from build123d import *

# Parameters (mm, degrees)
SKETCH_1_R          = 2.5
EXTRUDE_1_DEPTH     = 47
EXTRUDE_START       = 47
SKETCH_2_R          = 4
EXTRUDE_2_DEPTH     = 49
EXTRUDE_START_2     = 96
SKETCH_3_R          = 5
EXTRUDE_3_DEPTH     = 3.5
EXTRUDE_START_3     = 99.5
SKETCH_4_R          = 4
EXTRUDE_4_DEPTH     = 18
EXTRUDE_START_4     = 2.2
EXTRUDE_5_DEPTH     = 3
CHAMFER_1_SIZE      = 0.25
CHAMFER_2_SIZE      = 0.1
CUT_EXTRUDE_START   = 117.5
SKETCH_6_R          = 1.5
CUT_EXTRUDE_1_DEPTH = 10


with BuildPart() as part:
    # 草图1 → 凸台-拉伸1 (new body)
    with BuildSketch(Plane(origin=(0, 0, 0), x_dir=(1, 0, 0), z_dir=(0, 1, 0))):
        with Locations(Location((0, 0, 0), (0, 0, 270))):
            Circle(SKETCH_1_R)
    extrude(amount=EXTRUDE_1_DEPTH)

    # 草图2 → 凸台-拉伸2 (add)
    with BuildSketch(Plane(origin=(0, 0, 0), x_dir=(1, 0, 0), z_dir=(0, 1, 0)).offset(EXTRUDE_START)):
        with Locations(Location((0, 0, 0), (0, 0, 270))):
            Circle(SKETCH_2_R)
    extrude(amount=EXTRUDE_2_DEPTH)

    # 草图3 → 凸台-拉伸3 (add)
    with BuildSketch(Plane(origin=(0, 0, 0), x_dir=(1, 0, 0), z_dir=(0, 1, 0)).offset(EXTRUDE_START_2)):
        with Locations(Location((0, 0, 0), (0, 0, 270))):
            Circle(SKETCH_3_R)
    extrude(amount=EXTRUDE_3_DEPTH)

    # 草图4 → 凸台-拉伸4 (add)
    with BuildSketch(Plane(origin=(0, 0, 0), x_dir=(1, 0, 0), z_dir=(0, 1, 0)).offset(EXTRUDE_START_3)):
        with Locations(Location((0, 0, 0), (0, 0, 270))):
            Circle(SKETCH_4_R)
    extrude(amount=EXTRUDE_4_DEPTH)

    # 草图11 → 凸台-拉伸5 (add)
    with BuildSketch(Plane.XY.offset(EXTRUDE_START_4)):
        with BuildLine():
            Line((-1.5, 103), (-1.5, 114))
            ThreePointArc((-1.5, 114), (0, 115.5), (1.5, 114))
            Line((1.5, 114), (1.5, 103))
            ThreePointArc((1.5, 103), (0, 101.5), (-1.5, 103))
        make_face()
    extrude(amount=EXTRUDE_5_DEPTH)

    # 倒角1
    chamfer_1_edges = [part.edges().sort_by_distance(p)[0] for p in [
        (0, 117.5, -4),
        (0, 0, -2.5),
    ]]
    chamfer(chamfer_1_edges, length=CHAMFER_1_SIZE)

    # 倒角2
    chamfer_2_edges = [part.edges().sort_by_distance(p)[0] for p in [
        (0, 101.5, 5.2),
        (1.5, 108.5, 5.2),
        (0, 115.5, 5.2),
        (-1.5, 108.5, 5.2),
    ]]
    chamfer(chamfer_2_edges, length=CHAMFER_2_SIZE)

    # 草图6 → 切除-拉伸1 (cut)
    with BuildSketch(Plane(origin=(0, 0, 0), x_dir=(1, 0, 0), z_dir=(0, 1, 0)).offset(CUT_EXTRUDE_START)):
        with Locations(Location((0, 0, 0), (0, 0, 270))):
            Circle(SKETCH_6_R)
    extrude(amount=-CUT_EXTRUDE_1_DEPTH, mode=Mode.SUBTRACT)


solid = part.part
Source: CAD feature listing. Evaluate the final solid. Frame: model axes, mm. A direction names the side the tool comes from. Round coordinates to 2 decimals unless told otherwise and drop trailing zeros. Loops run counter-clockwise (first coordinate to the right, second up) from the corner with the lowest first, then second, coordinate; pieces in that order, holes last. Notation, with made-up numbers: (-33, -8.5) -> (-14, -8.5) arc R10 cw to (-14, 5.5) -> close; hole circle Ø10 at (1.25, -19.5). An arc over 180 degrees is marked (long way). Answer as a JSON object with one key per item and string values. Group by question number.
Q1. Section query A-A (z = 0). Output: boundary loops of the cut face in (x, y), plus the area to 3 significant figures.
Q2. Contact query for flat-ended pins moving along their axis: P1, Ø1.5, axis at x = -2.5, z = 2, coming from the -Y side; P2, Ø1.5, axis at x = 3.5, y = 34.5, coming from the -Z side; P3, Ø5, axis at x = 1.5, y = 37.5, coming from the -Z side; P4, Ø2.5, axis at x = 0, z = 0, coming from the +Y side. Output: stop coordinate, or through.
Q3. Access query for faces 5 (the flat face through (2, 47, 2)), 6 (the cylindrical face through (0.45, 112.57, 1.43)), 7 (the flat face through (-2, 117.5, 0)). Directions: +Z, -Z, +X, -X, +Y, -Y. A direction counts if a zero-diameter tool reaches every point of the face in a straight line with its end or side. Return the directions, or none.
Q4. Ray query, line 1 (X direction, y = 115.25, z = 0); line 2 (Y direction, x = -0.5, z = 0.25); line 3 (Y direction, x = 4.5, z = 0.75). Return the intervals inside material, ascending. Write a range as from..to.
Q5. Section query C-C (y = 16.5). Output: boundary loops of the cut face in (x, z), plus the area to 3 significant figures.
Q6. Section query D-D (y = 52). Output: boundary loops of the cut face in (x, z).
Q7. Mould query, pull axis Z, two halves, no side actions, for faces 1 (the flat face through (0, 107.5, 0)), 2 (the flat face through (0, 0, 0)), 3 (the flat face through (0, 109, 5.2)), 4 (the cylindrical face through (-4.88, 97.73, -1.08)). Classes: pulls with the +Z half, pulls with the -Z half, needs draft (parallel to the pull), parting line crosses it, or undercut.
Completed:
{
 "1": {"outline": "(-5, 96) -> (-4, 96) -> (-4, 47) -> (-2.5, 47) -> (-2.5, 0.25) -> (-2.25, 0) -> (2.25, 0) -> (2.5, 0.25) -> (2.5, 47) -> (4, 47) -> (4, 96) -> (5, 96) -> (5, 99.5) -> (4, 99.5) -> (4, 117.25) -> (3.75, 117.5) -> (1.5, 117.5) -> (1.5, 107.5) -> (-1.5, 107.5) -> (-1.5, 117.5) -> (-3.75, 117.5) -> (-4, 117.25) -> (-4, 99.5) -> (-5, 99.5) -> close", "area": "776 mm²"},
 "2": {"P1": "y = 0.2", "P2": "through", "P3": "z = -2.5", "P4": "y = 107.5"},
 "3": {"face 5": "-Y", "face 6": "+Y", "face 7": "+Z, -Z, +X, -X, +Y"},
 "4": {"line 1": "-4..-1.5, 1.5..4", "line 2": "0..107.5", "line 3": "96..99.5"},
 "5": {"outline": "circle Ø5 at (0, 0)", "area": "19.6 mm²"},
 "6": {"outline": "circle Ø8 at (0, 0)"},
 "7": {"face 1": "undercut", "face 2": "needs draft", "face 3": "pulls with the +Z half", "face 4": "parting line crosses it"}
}
